Part model, mm, in its own coordinate system. Face numbers are marked on the shaded views. A direction names the side the tool comes from. Round coordinates to 2 decimals unless told otherwise and drop trailing zeros. Loops run counter-clockwise (first coordinate to the right, second up) from the corner with the lowest first, then second, coordinate; pieces in that order, holes last.
1) Drop flat-ended pins along their axis: P1, Ø5, axis at x = -77.5, z = 15, coming from the -Y side; P2, Ø16, axis at x = 38.5, y = -15, coming from the +Z side; P3, Ø12, axis at x = -29, z = 31, coming from the +Y side; P4, Ø1.8, axis at x = 76.5, z = 14, coming from the +Y side. Give the stop position or say it passes through.
2) Band-saw the part on A-A, the plane y = 18.6. Write the cut outline in (x, z).
3) Band-saw the part on C-C, the plane z = 20.5. Write the cut outline in (x, y).
4) Probe line 1 (Y direction, x = -87.3, z = 12.5); line 2 (Z direction, x = 76.5, y = -1.15); line 3 (X direction, y = 31.5, z = 7). List the from-to ranges inside material, lowest first.
5) Band-saw the part on D-D, the plane x = 57.5. Write the cut outline in (y, z), then the cut area to 3 significant figures.
6) Mould opens along X. For the marked faces 3, 4 and 5 say: +X half, -X half, draft (parallel to the pull), parting line (faces both ways), or undercut.
7) 3-axis set-ups, long thin cutter, end or side, ignore diameter. For the marked faces 1 and 2: which of +Z, -Z, +X, -X, +Y, -Y reach the whole face in a straight line?
8) Band-saw the part on B-B, the plane x = 18.5. Write the cut outline in (y, z).
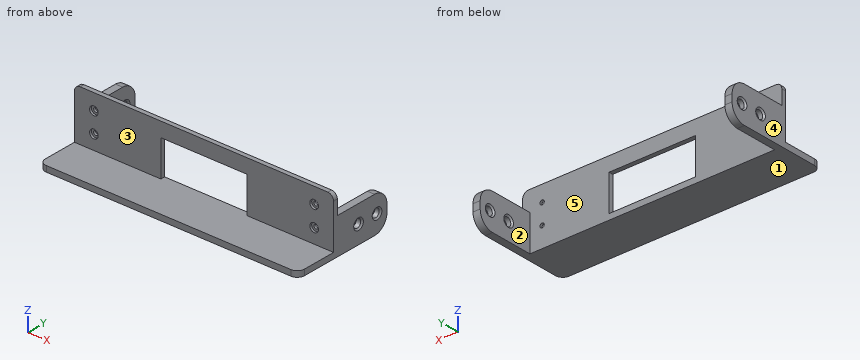
from build123d import *

# Parameters (mm, degrees)
SKETCH_1_W               = 180
SKETCH_1_H               = 60
EXTRUDE_1_DEPTH          = 4
SKETCH_2_W               = 180
SKETCH_2_H               = 3
EXTRUDE_2_DEPTH          = 35
SKETCH_3_R               = 1.5
CUT_EXTRUDE_1_DEPTH      = 50
FILLET_3_R               = 4
SKETCH_6_R               = 3
CUT_EXTRUDE_4_DEPTH      = 1.5
SKETCH_7_W               = 60
SKETCH_7_H               = 25
CUT_EXTRUDE_5_DEPTH      = 10
CUT_EXTRUDE_6_DEPTH      = 102.118742081
CUT_EXTRUDE_6_DEPTH_BACK = 102.118742081
SKETCH_8_W               = 180
SKETCH_8_H               = 28.5
SKETCH_9_W               = 25
SKETCH_9_H               = 40
EXTRUDE_3_DEPTH          = 5
CUT_EXTRUDE_7_DEPTH      = 189.794200123
CUT_EXTRUDE_7_DEPTH_BACK = 189.794200123
SKETCH_10_R              = 2.9
CHAMFER_2_SIZE           = 1
FILLET_4_R               = 5
CHAMFER_3_SIZE           = 1
FILLET_5_R               = 10
CHAMFER_4_SIZE           = 1


with BuildPart() as part:
    # 草图1 → 凸台-拉伸1 (new body)
    with BuildSketch(Plane.XY):
        Rectangle(SKETCH_1_W, SKETCH_1_H)
    extrude(amount=EXTRUDE_1_DEPTH)

    # 草图2 → 凸台-拉伸2 (add)
    with BuildSketch(Plane.XY.offset(4)):
        Rectangle(SKETCH_2_W, SKETCH_2_H)
    extrude(amount=EXTRUDE_2_DEPTH)

    # 草图3 → 切除-拉伸1 (cut)
    with BuildSketch(Plane.XZ.offset(1.5)):
        with Locations((-76.5, 28)):
            Circle(SKETCH_3_R)
        with Locations((-76.5, 14)):
            Circle(SKETCH_3_R)
        with Locations((76.5, 28)):
            Circle(SKETCH_3_R)
        with Locations((76.5, 14)):
            Circle(SKETCH_3_R)
    extrude(amount=-CUT_EXTRUDE_1_DEPTH, mode=Mode.SUBTRACT)

    # 圆角3
    fillet_3_edges = [part.edges().sort_by_distance(p)[0] for p in [
        (-90, 0, 39),
        (90, 0, 39),
    ]]
    fillet(fillet_3_edges, radius=FILLET_3_R)

    # 草图6 → 切除-拉伸4 (cut)
    with BuildSketch(Plane.XZ.offset(1.5)):
        with Locations((-76.5, 28)):
            Circle(SKETCH_6_R)
        with Locations((-76.5, 14)):
            Circle(SKETCH_6_R)
        with Locations((76.5, 28)):
            Circle(SKETCH_6_R)
        with Locations((76.5, 14)):
            Circle(SKETCH_6_R)
    extrude(amount=-CUT_EXTRUDE_4_DEPTH, mode=Mode.SUBTRACT)

    # 草图7 → 切除-拉伸5 (cut)
    with BuildSketch(Plane(origin=(0, 1.5, 0), x_dir=(1, 0, 0), z_dir=(0, 1, 0))):
        with Locations((0, -16.5)):
            Rectangle(SKETCH_7_W, SKETCH_7_H)
    extrude(amount=-CUT_EXTRUDE_5_DEPTH, mode=Mode.SUBTRACT)

    # 草图8 → 切除-拉伸6 (cut, two sides: drawn at the far end of the back side and taken through both)
    with BuildSketch(Plane.XY.offset(4).offset(-CUT_EXTRUDE_6_DEPTH_BACK)):
        with Locations((0, 15.75)):
            Rectangle(SKETCH_8_W, SKETCH_8_H)
    extrude(amount=CUT_EXTRUDE_6_DEPTH + CUT_EXTRUDE_6_DEPTH_BACK, mode=Mode.SUBTRACT)

    # 草图9 → 凸台-拉伸3 (add)
    with BuildSketch(Plane(origin=(90, 0, 0), x_dir=(0, 0, -1), z_dir=(1, 0, 0))):
        with Locations((-12.5, 21.5)):
            Rectangle(SKETCH_9_W, SKETCH_9_H)
    extrude_3 = extrude(amount=-EXTRUDE_3_DEPTH)

    # 镜向1: 凸台-拉伸3 across plane
    add(extrude_3.mirror(Plane(origin=(0, 0, 0), x_dir=(0, 0, 1), z_dir=(1, 0, 0))))

    # 草图10 → 切除-拉伸7 (cut, two sides: drawn at the far end of the back side and taken through both)
    with BuildSketch(Plane(origin=(90, 0, 0), x_dir=(0, 0, -1), z_dir=(1, 0, 0)).offset(-CUT_EXTRUDE_7_DEPTH_BACK)):
        with Locations(Location((-12.5, 33.5, 0), (0, 0, 90))):
            Circle(SKETCH_10_R)
        with Locations(Location((-12.5, 18.6, 0), (0, 0, 90))):
            Circle(SKETCH_10_R)
    extrude(amount=CUT_EXTRUDE_7_DEPTH + CUT_EXTRUDE_7_DEPTH_BACK, mode=Mode.SUBTRACT)

    # 倒角2
    chamfer_2_edges = [part.edges().sort_by_distance(p)[0] for p in [
        (85, 30.6, 12.5),
        (90, 30.6, 12.5),
        (-90, 30.6, 12.5),
        (-85, 30.6, 12.5),
    ]]
    chamfer(chamfer_2_edges, length=CHAMFER_2_SIZE)

    # 圆角4
    fillet_4_edges = [part.edges().sort_by_distance(p)[0] for p in [
        (90, -30, 2),
        (-90, -30, 2),
    ]]
    fillet(fillet_4_edges, radius=FILLET_4_R)

    # 倒角3
    chamfer_3_edges = [part.edges().sort_by_distance(p)[0] for p in [
        (90, 15.7, 12.5),
        (-90, 15.7, 12.5),
    ]]
    chamfer(chamfer_3_edges, length=CHAMFER_3_SIZE)

    # 圆角5
    fillet_5_edges = [part.edges().sort_by_distance(p)[0] for p in [
        (87.5, 41.5, 0),
        (87.5, 41.5, 25),
        (-87.5, 41.5, 0),
        (-87.5, 41.5, 25),
    ]]
    fillet(fillet_5_edges, radius=FILLET_5_R)

    # 倒角4
    chamfer_4_edges = [part.edges().sort_by_distance(p)[0] for p in [
        (85, 15.7, 12.5),
        (-85, 15.7, 12.5),
    ]]
    chamfer(chamfer_4_edges, length=CHAMFER_4_SIZE)


solid = part.part
Reported:
1. P1: stops at y = -1.5
1. P2: stops at z = 4
1. P3: stops at y = 1.5
1. P4: passes through
2. outline: (-90, 0) - (-85, 0) - (-85, 8.6) - (-86, 9.6) - (-89, 9.6) - (-90, 8.6) - close; (-90, 16.4) - (-89, 15.4) - (-86, 15.4) - (-85, 16.4) - (-85, 25) - (-90, 25) - close; (85, 0) - (90, 0) - (90, 8.6) - (89, 9.6) - (86, 9.6) - (85, 8.6) - close; (85, 16.4) - (86, 15.4) - (89, 15.4) - (90, 16.4) - (90, 25) - (85, 25) - close
3. outline: (-90, -1.5) - (-30, -1.5) - (-30, 1.5) - (-85, 1.5) - (-85, 39.85) - (-90, 39.85) - close; (30, -1.5) - (90, -1.5) - (90, 39.85) - (85, 39.85) - (85, 1.5) - (30, 1.5) - close
4. line 1: y = -1.5 to 15.7, 21.5 to 30.6, 36.4 to 41.5
4. line 2: z = 0 to 11, 17 to 25, 31 to 39
4. line 3: x = -90 to -85, 85 to 90
5. outline: (-30, 0) - (1.5, 0) - (1.5, 39) - (-1.5, 39) - (-1.5, 4) - (-30, 4) - close
5. area: 231 mm2
6. face 3: draft
6. face 4: -X half
6. face 5: undercut
7. face 1: -Z, +X, -X, +Y, -Y
7. face 2: +Z, -Z, +Y
8. outline: (-30, 0) - (1.5, 0) - (1.5, 4) - (-30, 4) - close; (-1.5, 29) - (1.5, 29) - (1.5, 39) - (-1.5, 39) - close
